Geometry check sheet. Reference: the model listing, model coordinates, mm. Round coordinates to 2 decimals unless told otherwise and drop trailing zeros. Order: outer loops, then holes, each group sorted by start corner. A loop starts at its lowest first (then second) coordinate and runs counter-clockwise, first axis right, second up.
(1) Go/stop test with flat-tipped pins: pin 1 (1.9 mm diameter, centred on x = 20, y = -22.5, fed in from -Z); pin 2 (1 mm diameter, centred on x = 21.5, z = 2, fed in from -Y); pin 3 (1.5 mm diameter, centred on y = 19.5, z = 1.5, fed in from +X). Record where each tip stops, or that it passes through.
(2) Sectioned sample at A-A (x = 20). Record the boundary of the cut face in (y, z), plus the area to 3 significant figures.
(3) Material ranges on line 1 along Y through (x, z) = (45, 0.6); line 2 along Y through (x, z) = (52.75, 1.9); line 3 along X through (y, z) = (-23.5, 2.8), recorded low to high.
(4) Sectioned sample at B-B (y = -1). Record the boundary of the cut face in (x, z), plus the area to 3 significant figures.
(5) Sectioned sample at C-C (x = 36.5). Record the boundary of the cut face in (y, z).
(6) Sectioned sample at D-D (y = 17.5). Record the boundary of the cut face in (x, z).
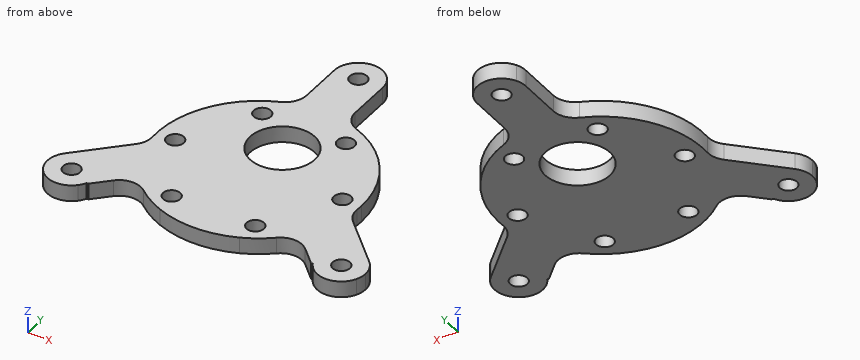
from build123d import *

# Parameters (mm, degrees)
SKETCH_1_R      = 1.6
SKETCH_1_R_2    = 6
EXTRUDE_1_DEPTH = 3
FILLET_1_R      = 4


with BuildPart() as part:
    # 草图1 → 凸台-拉伸1 (new body)
    # profile 1 of 13: a face of its own
    with BuildSketch(Plane.XY):
        with BuildLine():
            ThreePointArc((64, -7), (59.941552797, 4.736694594), (49.5, 11.459414942))
            ThreePointArc((49.5, 11.459414942), (45, 12), (40.5, 11.459414942))
            ThreePointArc((40.5, 11.459414942), (29.2006815, 3.553745068), (26.224418371, -9.911620598))
            ThreePointArc((26.224418371, -9.911620598), (27.583310363, -14.593347225), (30.0887682, -18.775192831))
            ThreePointArc((30.0887682, -18.775192831), (33.483334572, -22.111797293), (37.600675707, -24.5))
            Line((37.600675707, -24.5), (52.399324293, -24.5))
            ThreePointArc((52.399324293, -24.5), (56.516665428, -22.111797293), (59.9112318, -18.775192831))
            ThreePointArc((59.9112318, -18.775192831), (62.416689637, -14.593347225), (63.775581629, -9.911620598))
            ThreePointArc((63.775581629, -9.911620598), (63.943812327, -8.460128257), (64, -7))
        make_face()
        with Locations((37.25, -20.423393759)):
            Circle(SKETCH_1_R, mode=Mode.SUBTRACT)
        with Locations((52.75, -20.423393759)):
            Circle(SKETCH_1_R, mode=Mode.SUBTRACT)
        with Locations((29.5, -7)):
            Circle(SKETCH_1_R, mode=Mode.SUBTRACT)
        with Locations((60.5, -7)):
            Circle(SKETCH_1_R, mode=Mode.SUBTRACT)
        with Locations((45, 0)):
            Circle(SKETCH_1_R_2, mode=Mode.SUBTRACT)
        with Locations((37.25, 6.423393759)):
            Circle(SKETCH_1_R, mode=Mode.SUBTRACT)
        with Locations((52.75, 6.423393759)):
            Circle(SKETCH_1_R, mode=Mode.SUBTRACT)
    # profile 2 of 13: a face of its own
    with BuildSketch(Plane.XY):
        with BuildLine():
            ThreePointArc((30.0887682, -18.775192831), (27.583310363, -14.593347225), (26.224418371, -9.911620598))
            Line((26.224418371, -9.911620598), (16.818019485, -19.318019485))
            ThreePointArc((16.818019485, -19.318019485), (21.722075446, -18.342542104), (24.5, -22.5))
            Line((24.5, -22.5), (24.5, -24.363961031))
            Line((24.5, -24.363961031), (30.0887682, -18.775192831))
        make_face()
    # profile 3 of 13: a face of its own
    with BuildSketch(Plane.XY):
        with BuildLine():
            ThreePointArc((24.5, -22.5), (21.722075446, -18.342542104), (16.818019485, -19.318019485))
            ThreePointArc((16.818019485, -19.318019485), (15.842542104, -20.777924554), (15.5, -22.5))
            ThreePointArc((15.5, -22.5), (15.61878556, -23.527112473), (15.968871126, -24.5))
            Line((15.968871126, -24.5), (24.031128874, -24.5))
            ThreePointArc((24.031128874, -24.5), (24.38121444, -23.527112473), (24.5, -22.5))
        make_face()
        with Locations((20, -22.5)):
            Circle(SKETCH_1_R, mode=Mode.SUBTRACT)
    # profile 4 of 13: a face of its own
    with BuildSketch(Plane.XY):
        with BuildLine():
            Line((24.031128874, -24.5), (15.968871126, -24.5))
            ThreePointArc((15.968871126, -24.5), (19.272310012, -26.940773275), (23.181980515, -25.681980515))
            ThreePointArc((23.181980515, -25.681980515), (23.654655422, -25.125546372), (24.031128874, -24.5))
        make_face()
    # profile 5 of 13: a face of its own
    with BuildSketch(Plane.XY):
        with BuildLine():
            ThreePointArc((66.818019485, -25.681980515), (70.727689988, -26.940773275), (74.031128874, -24.5))
            Line((74.031128874, -24.5), (65.968871126, -24.5))
            ThreePointArc((65.968871126, -24.5), (66.345344578, -25.125546372), (66.818019485, -25.681980515))
        make_face()
    # profile 6 of 13: a face of its own
    with BuildSketch(Plane.XY):
        with BuildLine():
            ThreePointArc((65.5, -22.5), (68.277924554, -18.342542104), (73.181980515, -19.318019485))
            Line((73.181980515, -19.318019485), (63.775581629, -9.911620598))
            ThreePointArc((63.775581629, -9.911620598), (62.416689637, -14.593347225), (59.9112318, -18.775192831))
            Line((59.9112318, -18.775192831), (65.5, -24.363961031))
            Line((65.5, -24.363961031), (65.5, -22.5))
        make_face()
    # profile 7 of 13: a face of its own
    with BuildSketch(Plane.XY):
        with BuildLine():
            Line((49.5, 11.459414942), (49.5, 22.5))
            ThreePointArc((49.5, 22.5), (45, 18), (40.5, 22.5))
            Line((40.5, 22.5), (40.5, 11.459414942))
            ThreePointArc((40.5, 11.459414942), (45, 12), (49.5, 11.459414942))
        make_face()
    # profile 8 of 13: a face of its own
    with BuildSketch(Plane.XY):
        with BuildLine():
            ThreePointArc((49.5, 22.5), (49.38121444, 23.527112473), (49.031128874, 24.5))
            Line((49.031128874, 24.5), (40.968871126, 24.5))
            ThreePointArc((40.968871126, 24.5), (40.61878556, 23.527112473), (40.5, 22.5))
            ThreePointArc((40.5, 22.5), (45, 18), (49.5, 22.5))
        make_face()
        with Locations((45, 22.5)):
            Circle(SKETCH_1_R, mode=Mode.SUBTRACT)
    # profile 9 of 13: a face of its own
    with BuildSketch(Plane.XY):
        with BuildLine():
            Line((40.968871126, 24.5), (49.031128874, 24.5))
            ThreePointArc((49.031128874, 24.5), (45, 27), (40.968871126, 24.5))
        make_face()
    # profile 10 of 13: a face of its own
    with BuildSketch(Plane.XY):
        with BuildLine():
            Line((24.5, -24.363961031), (24.5, -22.5))
            ThreePointArc((24.5, -22.5), (24.38121444, -23.527112473), (24.031128874, -24.5))
            Line((24.031128874, -24.5), (24.363961031, -24.5))
            Line((24.363961031, -24.5), (24.5, -24.363961031))
        make_face()
    # profile 11 of 13: a face of its own
    with BuildSketch(Plane.XY):
        with BuildLine():
            Line((65.636038969, -24.5), (65.968871126, -24.5))
            ThreePointArc((65.968871126, -24.5), (65.61878556, -23.527112473), (65.5, -22.5))
            Line((65.5, -22.5), (65.5, -24.363961031))
            Line((65.5, -24.363961031), (65.636038969, -24.5))
        make_face()
    # profile 12 of 13: a face of its own
    with BuildSketch(Plane.XY):
        with BuildLine():
            Line((65.968871126, -24.5), (74.031128874, -24.5))
            ThreePointArc((74.031128874, -24.5), (74.38121444, -23.527112473), (74.5, -22.5))
            ThreePointArc((74.5, -22.5), (74.157457896, -20.777924554), (73.181980515, -19.318019485))
            ThreePointArc((73.181980515, -19.318019485), (68.277924554, -18.342542104), (65.5, -22.5))
            ThreePointArc((65.5, -22.5), (65.61878556, -23.527112473), (65.968871126, -24.5))
        make_face()
        with Locations((70, -22.5)):
            Circle(SKETCH_1_R, mode=Mode.SUBTRACT)
    # profile 13 of 13: a face of its own
    with BuildSketch(Plane.XY):
        with BuildLine():
            ThreePointArc((37.600675707, -24.5), (45, -26), (52.399324293, -24.5))
            Line((52.399324293, -24.5), (37.600675707, -24.5))
        make_face()
    extrude(amount=EXTRUDE_1_DEPTH)

    # 圆角1
    fillet_1_edges = [part.edges().sort_by_distance(p)[0] for p in [
        (59.9112318, -18.775192831, 1.5),
        (30.0887682, -18.775192831, 1.5),
        (26.224418371, -9.911620598, 1.5),
        (40.5, 11.459414942, 1.5),
        (49.5, 11.459414942, 1.5),
        (63.775581629, -9.911620598, 1.5),
    ]]
    fillet(fillet_1_edges, radius=FILLET_1_R)


solid = part.part
Answer below:
1. pin 1: passes through
1. pin 2: stops at y = -26.89
1. pin 3: stops at x = 49.5
2. outline: (-27, 0) - (-24.1, 0) - (-24.1, 3) - (-27, 3) - close; (-20.9, 0) - (-16.14, 0) - (-16.14, 3) - (-20.9, 3) - close
2. area: 23.0 mm2
3. line 1: y = -26 to -6, 6 to 20.9, 24.1 to 27
3. line 2: y = -24.35 to -22.02, -18.82 to 4.82, 8.02 to 10.35
3. line 3: x = 15.61 to 18.75, 21.25 to 25.36, 35.58 to 54.42, 64.64 to 68.75, 71.25 to 74.39
4. outline: (26.97, 0) - (39.08, 0) - (39.08, 3) - (26.97, 3) - close; (50.92, 0) - (63.03, 0) - (63.03, 3) - (50.92, 3) - close
4. area: 72.7 mm2
5. outline: (-23.99, 0) - (-21.84, 0) - (-21.84, 3) - (-23.99, 3) - close; (-19.01, 0) - (5.01, 0) - (5.01, 3) - (-19.01, 3) - close; (7.84, 0) - (9.99, 0) - (9.99, 3) - (7.84, 3) - close
6. outline: (40.5, 0) - (49.5, 0) - (49.5, 3) - (40.5, 3) - close
